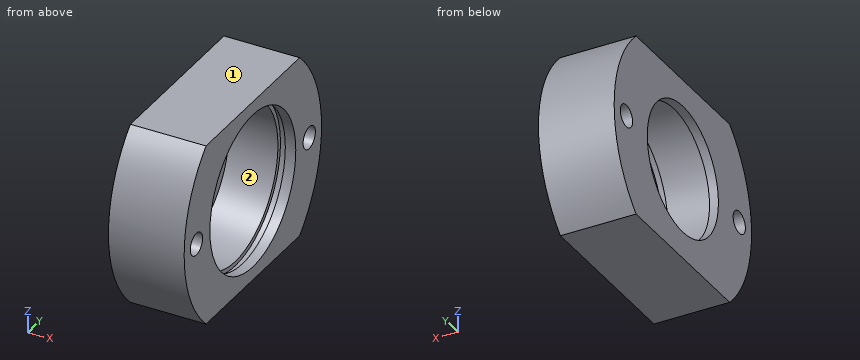
from build123d import *

# Parameters (mm, degrees)
CUT_EXTRUDE1_DEPTH = 44.092922853
TAPPED_HOLE1_D     = 5


with BuildPart() as part:
    # Sketch1 → Revolve1 (revolve)
    with BuildSketch(Plane.XY, mode=Mode.PRIVATE) as revolve1_sk:
        Polygon((0, 28), (17, 28), (17, 17.5), (14.65, 17.5), (14.65, 18.5), (13, 18.5), (13, 17.5), (2, 17.5), (2, 14.5), (0, 14.5), align=None)
    revolve(revolve1_sk.sketch.rotate(Axis((0, 0, 0), (1, 0, 0)), 90), axis=Axis((0, 0, 0), (1, 0, 0)))

    # Sketch2 → Cut-Extrude1 (cut, through all)
    with BuildSketch(Plane(origin=(17, 0, 0), x_dir=(0, 0, -1), z_dir=(1, 0, 0))):
        with BuildLine():
            Line((-20.5, 19.072231123), (-20.5, -19.072231123))
            ThreePointArc((-20.5, -19.072231123), (-28, 0), (-20.5, 19.072231123))
        make_face()
        with BuildLine():
            Line((20.5, 19.072231123), (20.5, -19.072231123))
            ThreePointArc((20.5, -19.072231123), (28, 0), (20.5, 19.072231123))
        make_face()
    extrude(amount=-CUT_EXTRUDE1_DEPTH, mode=Mode.SUBTRACT)

    # Tapped Hole1 (through all)
    with Locations(Plane(origin=(17, 0, 0), x_dir=(0, 0, -1), z_dir=(1, 0, 0))):
        with Locations((0, 23), (0, -23)):
            Hole(TAPPED_HOLE1_D / 2)


solid = part.part
Work out the finished part from the listing and answer in its coordinate system (mm). Face numbers are marked on the shaded views. A direction names the side the tool comes from. Give positions to 0.01 mm unless a question says otherwise; leave off trailing zeros. Loops run counter-clockwise (first coordinate to the right, second up) from the corner with the lowest first, then second, coordinate; pieces in that order, holes last. Notation, with made-up numbers: M 22.5,-28.75 L 76.5,-28.75 A14 ccw 76.5,-3.75 Z; hole C 30.5,-6 d8. An arc over 180 degrees is marked long. Use CSV: the item, a comma, the result in double quotes.
1) Consider L1, parallel to Y at x = 13.55, z = 0; L2, parallel to Y at x = 4.5, z = 0; L3, parallel to X at y = 8.5, z = 12.5. Determine where each line is inside the solid, lowest interval first.
Answer:
L1,"-28 to -25.5, -20.5 to -18.5, 18.5 to 20.5, 25.5 to 28"
L2,"-28 to -25.5, -20.5 to -17.5, 17.5 to 20.5, 25.5 to 28"
L3,"0 to 2"
2) Find section D-D on z = 10. Write down the section's boundary in (x, y).
Answer:
outline,"M 0,-26.15 L 17,-26.15 L 17,-14.36 L 14.65,-14.36 L 14.65,-15.56 L 13,-15.56 L 13,-14.36 L 2,-14.36 L 2,-10.5 L 0,-10.5 Z; M 0,10.5 L 2,10.5 L 2,14.36 L 13,14.36 L 13,15.56 L 14.65,15.56 L 14.65,14.36 L 17,14.36 L 17,26.15 L 0,26.15 Z"
3) Given P1, Ø5, axis at x = 3.5, z = 1, coming from the -Y side; P2, Ø4, axis at y = -23, z = 0, coming from the -X side; P3, Ø10, axis at x = 11, z = 15, coming from the +Y side; P4, Ø8, axis at x = 11, y = -22, coming from the -Z side, each flat-ended and moving along its own axis, determine where each tip first touches the part or whether it passes through.
Answer:
P1,"y = -28"
P2,"through"
P3,"y = 26.15"
P4,"z = -20.5"
4) Find section B-B on y = 0. Write down the section's boundary in (x, z), plus the area to 3 significant figures.
Answer:
outline,"M 0,-20.5 L 17,-20.5 L 17,-17.5 L 14.65,-17.5 L 14.65,-18.5 L 13,-18.5 L 13,-17.5 L 2,-17.5 L 2,-14.5 L 0,-14.5 Z; M 0,14.5 L 2,14.5 L 2,17.5 L 13,17.5 L 13,18.5 L 14.65,18.5 L 14.65,17.5 L 17,17.5 L 17,20.5 L 0,20.5 Z"
area,"111 mm^2"
5) Which of the six approach directions +Z, -Z, +X, -X, +Y, -Y give full straight-line access (tool end or side, diameter ignored) to the marked faces 1 and 2?
Answer:
face 1,"+Z, +X, -X, +Y, -Y"
face 2,"+X"
6) Find section C-C on x = 7.25. Write down the section's boundary in (y, z), plus the area to 3 significant figures.
Answer:
outline,"M -19.07,-20.5 L 19.07,-20.5 A28 ccw 19.07,20.5 L -19.07,20.5 A28 ccw Z; hole C -23,0 d5; hole C 0,0 d35; hole C 23,0 d5"
area,"1,070 mm^2"
7) Find section A-A on z = 0. Write down the section's boundary in (x, y), plus the area to 3 significant figures.
Answer:
outline,"M 0,-28 L 17,-28 L 17,-25.5 L 0,-25.5 Z; M 0,-20.5 L 17,-20.5 L 17,-17.5 L 14.65,-17.5 L 14.65,-18.5 L 13,-18.5 L 13,-17.5 L 2,-17.5 L 2,-14.5 L 0,-14.5 Z; M 0,14.5 L 2,14.5 L 2,17.5 L 13,17.5 L 13,18.5 L 14.65,18.5 L 14.65,17.5 L 17,17.5 L 17,20.5 L 0,20.5 Z; M 0,25.5 L 17,25.5 L 17,28 L 0,28 Z"
area,"196 mm^2"
